Autodesk Fusion 360 part; units mm, degrees
sketch "Sketch1" plane through (0, 0, 0) normal (0, 1, 0) x (1, 0, 0)
  line L0 (0, 0) -> (20.25, 0)
  line L1 (20.25, 0) -> (20.25, 2.5)
  line L2 (20.25, 2.5) -> (0, 2.5)
  line L3 (0, 2.5) -> (0, 0)
  line L4 (0, 0) -> (1.25, 0)
  line L5 (1.25, 0) -> (1.25, 1.25)
  line L6 (1.5, 1) -> (1, 1)
  line L7 (1, 1) -> (1, 1.5)
  line L8 (1, 1.5) -> (1.5, 1.5)
  line L9 (1.5, 1.5) -> (1.5, 1)
  line L10 (1.5, 1) -> (1, 1.5) construction
  line L11 (1, 1) -> (1.5, 1.5) construction
  line L12 (1.25, 1.25) -> (3.75, 1.25)
  line L13 (4, 1) -> (3.5, 1)
  line L14 (3.5, 1) -> (3.5, 1.5)
  line L15 (3.5, 1.5) -> (4, 1.5)
  line L16 (4, 1.5) -> (4, 1)
  line L17 (4, 1) -> (3.5, 1.5) construction
  line L18 (3.5, 1) -> (4, 1.5) construction
  line L19 (3.75, 1.25) -> (6.25, 1.25)
  line L20 (6.5, 1) -> (6, 1)
  line L21 (6, 1) -> (6, 1.5)
  line L22 (6, 1.5) -> (6.5, 1.5)
  line L23 (6.5, 1.5) -> (6.5, 1)
  line L24 (6.5, 1) -> (6, 1.5) construction
  line L25 (6, 1) -> (6.5, 1.5) construction
  line L26 (6.25, 1.25) -> (8.75, 1.25)
  line L27 (9, 1) -> (8.5, 1)
  line L28 (8.5, 1) -> (8.5, 1.5)
  line L29 (8.5, 1.5) -> (9, 1.5)
  line L30 (9, 1.5) -> (9, 1)
  line L31 (9, 1) -> (8.5, 1.5) construction
  line L32 (8.5, 1) -> (9, 1.5) construction
  line L33 (8.75, 1.25) -> (11.25, 1.25)
  line L34 (11.5, 1.5) -> (11, 1.5)
  line L35 (11, 1.5) -> (11, 1)
  line L36 (11, 1) -> (11.5, 1)
  line L37 (11.5, 1) -> (11.5, 1.5)
  line L38 (11.5, 1.5) -> (11, 1) construction
  line L39 (11, 1.5) -> (11.5, 1) construction
  line L40 (11.25, 1.25) -> (13.75, 1.25)
  line L41 (14, 1.5) -> (13.5, 1.5)
  line L42 (13.5, 1.5) -> (13.5, 1)
  line L43 (13.5, 1) -> (14, 1)
  line L44 (14, 1) -> (14, 1.5)
  line L45 (14, 1.5) -> (13.5, 1) construction
  line L46 (13.5, 1.5) -> (14, 1) construction
  line L47 (13.75, 1.25) -> (16.25, 1.25)
  line L48 (16.5, 1) -> (16, 1)
  line L49 (16, 1) -> (16, 1.5)
  line L50 (16, 1.5) -> (16.5, 1.5)
  line L51 (16.5, 1.5) -> (16.5, 1)
  line L52 (16.5, 1) -> (16, 1.5) construction
  line L53 (16, 1) -> (16.5, 1.5) construction
  line L54 (16.25, 1.25) -> (18.75, 1.25)
  line L55 (19, 1) -> (18.5, 1)
  line L56 (18.5, 1) -> (18.5, 1.5)
  line L57 (18.5, 1.5) -> (19, 1.5)
  line L58 (19, 1.5) -> (19, 1)
  line L59 (19, 1) -> (18.5, 1.5) construction
  line L60 (18.5, 1) -> (19, 1.5) construction
  point P0 (1.25, 1.25)
  point P1 (3.75, 1.25)
  point P2 (6.25, 1.25)
  point P3 (8.75, 1.25)
  point P4 (11.25, 1.25)
  point P5 (13.75, 1.25)
  point P6 (16.25, 1.25)
  point P7 (18.75, 1.25)
  dimension "d1" = 20.25
  dimension "d2" = 0.5
  dimension "d3" = 0.5
  dimension "d4" = 0.5
  dimension "d5" = 0.5
  dimension "d6" = 2.5
  dimension "d7" = 0.5
  dimension "d8" = 0.5
  dimension "d9" = 0.5
  dimension "d10" = 0.5
  dimension "d11" = 2.5
  dimension "d12" = 0.5
  dimension "d13" = 0.5
  dimension "d14" = 2.5
  dimension "d15" = 0.5
  dimension "d16" = 0.5
  dimension "d17" = 2.5
  dimension "d18" = 0.5
  dimension "d19" = 0.5
  dimension "d24" = 2.5
  dimension "d25" = 1.25
  dimension "d26" = 1.25
  dimension "d27" = 2.5
  dimension "d28" = 2.5
  dimension "d29" = 2.5
extrude "Extrude1" add sketch "Sketch1" along normal blind 2.5 makes body 1
extrude "Extrude2" add sketch "Sketch1" along normal blind 8.5 separate body contours L55 L56 L57 L58 | L47 L49 L50 L51 L54 | L47 L48 L49 L51 L54 | L40 L41 L42 L44 L47 | L40 L42 L43 L44 L47 | L33 L34 L35 L37 L40 | L33 L35 L36 L37 L40 | L26 L28 L29 L30 L33 | L26 L27 L28 L30 L33 | L19 L21 L22 L23 L26 | L19 L20 L21 L23 L26 | L12 L14 L15 L16 L19 | L12 L13 L14 L16 L19 | L5 L6 L7 L8 L9 L12 | L5 L6 L9 L12 makes body 2 at (13.6667, 2.8333, -1) makes body 3 at (3.6667, 2.8333, -1.5) makes body 4 at (6, 2.8333, -1.1667) makes body 5 at (16.5, 2.8333, -1.3333) makes body 6 at (11.3333, 2.8333, -1.5) makes body 7 at (1, 2.8333, -1.1667) makes body 8 at (8.5, 2.8333, -1.1667) makes body 9 at (18.5, 2.8333, -1.1667)
extrude "Extrude3" add sketch "Sketch1" against normal blind 2.5 contours L55 L56 L57 L58 | L47 L49 L50 L51 L54 | L47 L48 L49 L51 L54 | L40 L41 L42 L44 L47 | L40 L42 L43 L44 L47 | L33 L34 L35 L37 L40 | L33 L35 L36 L37 L40 | L26 L28 L29 L30 L33 | L26 L27 L28 L30 L33 | L19 L21 L22 L23 L26 | L19 L20 L21 L23 L26 | L12 L14 L15 L16 L19 | L12 L13 L14 L16 L19 | L5 L6 L7 L8 L9 L12 | L5 L6 L9 L12 bodies 2 1 3 4 5 6 7 8 9
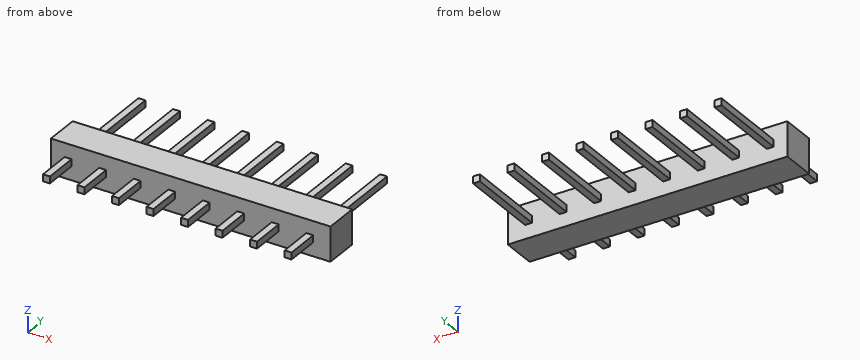
Check sheet for the modelled part. Datum: model origin and axes. Units: mm. Give positions to 0.01 mm unless a question says otherwise; leave off trailing zeros. Loops run counter-clockwise (first coordinate to the right, second up) from the corner with the lowest first, then second, coordinate; pieces in that order, holes last. Notation, with made-up numbers: M 8,-28.5 L 45,-28.5 A29 cw 45,8.5 Z; hole C -22.75,29.25 d6. An arc over 180 degrees is marked long. Return JSON: item names as keys, results as strings. Group by question number.
1. Cross-section at B-B on x = 14.25. Record the boundary of the cut face in (y, z).
2. Go/stop test with flat-tipped pins: pin 1 (2 mm diameter, centred on x = 6, y = 5, fed in from -Z); pin 2 (0.8 mm diameter, centred on x = 10.5, z = -1, fed in from +Y); pin 3 (0.6 mm diameter, centred on y = -1.5, z = -1.5, fed in from +X). Record where each tip stops, or that it passes through.
3. Cross-section at A-A on y = 5.25. State how many separate pieces and enclosed holes the cut face has, plus the area to 3 significant figures.
4. Cross-section at C-C on z = -0.7. Record the boundary of the cut face in (x, y), plus the area to 3 significant figures.
5. Thickness scan on L1, parallel to Y at x = 6.5, z = -2.3; L2, parallel to Z at x = 1.25, y = 5.5. Record the ranges inside material, lowest first.
Return value:
{
 "1": {"outline": "M 0,-2.5 L 2.5,-2.5 L 2.5,0 L 0,0 Z"},
 "2": {"pin 1": "z = -1.5", "pin 2": "y = 2.5", "pin 3": "x = 19"},
 "3": {"separate pieces": "8", "enclosed holes": "0", "area": "2.00 mm^2"},
 "4": {"outline": "M 0,0 L 20.25,0 L 20.25,2.5 L 0,2.5 Z", "area": "50.6 mm^2"},
 "5": {"L1": "0 to 2.5", "L2": "-1.5 to -1"}
}
